```python
from build123d import *

# Parameters (mm, degrees)
BOSS_EXTRUDE1_DEPTH = 0.762


with BuildPart() as part:
    # Sketch1 → Boss-Extrude1 (new body)
    with BuildSketch(Plane(origin=(0, 0, 0), x_dir=(1, 0, 0), z_dir=(0, 1, 0))):
        with BuildLine():
            ThreePointArc((66.167, 0), (61.130337028, 25.321014669), (46.787134391, 46.787134391))
            ThreePointArc((46.787134391, 46.787134391), (40.500955106, 46.787134391), (40.500955106, 40.500955106))
            ThreePointArc((40.500955106, 40.500955106), (52.917047984, 21.918958956), (57.277, 0))
            ThreePointArc((57.277, 0), (61.722, -4.445), (66.167, 0))
        make_face()
        with BuildLine():
            ThreePointArc((65.151, 0), (60.191675423, 24.932208302), (46.068713901, 46.068713901))
            ThreePointArc((46.068713901, 46.068713901), (41.219375596, 46.068713901), (41.219375596, 41.219375596))
            ThreePointArc((41.219375596, 41.219375596), (53.855709589, 22.307765323), (58.293, 0))
            ThreePointArc((58.293, 0), (61.722, -3.429), (65.151, 0))
        make_face(mode=Mode.SUBTRACT)
    extrude(amount=BOSS_EXTRUDE1_DEPTH)


solid = part.part
```
Geometry check sheet. Reference: the model listing, model coordinates, mm. A direction names the side the tool comes from. Give positions to 0.01 mm unless a question says otherwise; leave off trailing zeros. Write each loop counter-clockwise with the first axis right and the second up, starting at its lowest first coordinate (ties: lowest second). Pieces come first, ordered by that corner, then holes. Notation, with made-up numbers: (53.5, -6) - (104.5, -6) arc R34 ccw to (104.5, 31) - close; hole circle Ø11 at (-36.5, -8.75). An arc over 180 degrees is marked (long way). Use a Markdown table: item, result.
Q1. Set-up check for faces 4 (the face through (53.6, 0.762, -21.9)), 5 (the face through (60.33, 0.38, -24.6)): record each of +Z, -Z, +X, -X, +Y, -Y from which the full face is reachable in a straight line by a thin tool's end or side.
Computed:
| item | result |
|---|---|
| face 4 | +Z, -Z, +X, -X, +Y |
| face 5 | +Y, -Y |
Q2. Section check B-B, the plane y = 0.45. Enter the section's corners in (x, z) (3 decimals), then the cut area to 3 significant figures.
Computed:
| item | result |
|---|---|
| outline | (40.501, -40.501) arc R4.445 ccw to (46.787, -46.787) arc R66.167 ccw to (66.167, 0) arc R4.445 ccw to (57.277, 0) arc R57.277 cw to start; hole (41.219, -41.219) arc R3.429 ccw to (46.069, -46.069) arc R65.151 ccw to (65.151, 0) arc R3.429 ccw to (58.293, 0) arc R58.293 cw to start |
| area | 124 mm² |
Q3. Section check A-A, the plane z = -40. Enter the section's corners in (x, y).
Computed:
| item | result |
|---|---|
| outline | (41, 0) - (42.4, 0) - (42.4, 0.76) - (41, 0.76) - close; (51.43, 0) - (52.71, 0) - (52.71, 0.76) - (51.43, 0.76) - close |
Q4. Draft check along X on faces 1 (the face through (40.571, 0.376, -46.855)), 2 (the face through (61.65, 0.38, 3.43)), 3 (the face through (52.8, 0.4, -22.2)). Enter one of: pulls with the +X half, pulls with the -X half, needs draft (parallel to the pull), parting line crosses it, or undercut.
Computed:
| item | result |
|---|---|
| face 1 | parting line crosses it |
| face 2 | undercut |
| face 3 | pulls with the -X half |
Q5. Section check C-C, the plane x = 48.5. Enter the section's corners in (y, z).
Computed:
| item | result |
|---|---|
| outline | (0, -45.01) - (0.76, -45.01) - (0.76, -43.5) - (0, -43.5) - close; (0, -32.34) - (0.76, -32.34) - (0.76, -30.47) - (0, -30.47) - close |
Q6. Thickness scan on L1, parallel to X at y = 0.35, z = -43.5; L2, parallel to Z at x = 51.75, y = 0.3; L3, parallel to Z at x = 51.5, y = 0.55. Record the ranges inside material, lowest first. Write a range as [from, to].
Computed:
| item | result |
|---|---|
| L1 | x = [39.2, 40.22], [48.5, 49.86] |
| L2 | z = [-41.23, -39.58], [-26.83, -24.55] |
| L3 | z = [-41.54, -39.9], [-27.31, -25.07] |
